Geometry: final body of the model. Coordinates: model frame, mm. Face numbers are marked on the shaded views. Coordinates: 2 decimals unless noted, no trailing zeros. Write each loop counter-clockwise with the first axis right and the second up, starting at its lowest first coordinate (ties: lowest second). Pieces come first, ordered by that corner, then holes. Notation, with made-up numbers: (89.5, 45) -> (148.5, 45) arc R25 cw to (148.5, 81) -> close; hole circle Ø9 at (-23, 47.25). An arc over 180 degrees is marked (long way). Answer as a JSON object with one key per item and string values. Group by question number.
```python
from build123d import *

# Parameters (mm, degrees)
F0_R     = 5
F1_DEPTH = 1
F3_DEPTH = 5
F4_W     = 11.32601
F4_H     = 3.74272
F5_DEPTH = 5
F6_R     = 2.25
F7_DEPTH = 3
F8_R     = 1
F9_DEPTH = 25


with BuildPart() as f1:
    # F0 (on Front) → F1 (new body)
    with BuildSketch(Plane.XZ):
        Circle(F0_R)
    extrude(amount=F1_DEPTH)

    # F2 (on face) → F3 (join)
    with BuildSketch(Plane.XZ.offset(1)):
        with BuildLine():
            ThreePointArc((0, -6), (4.242641, -4.242641), (6, 0))
            ThreePointArc((6, 0), (4.242641, 4.242641), (0, 6))
            ThreePointArc((0, 6), (-3.774917, 4.66369), (-5.868347, 1.25))
            Line((-5.868347, 1.25), (4, 1.25))
            Line((4, 1.25), (4, -1.25))
            Line((4, -1.25), (-5.868347, -1.25))
            ThreePointArc((-5.868347, -1.25), (-3.774917, -4.66369), (0, -6))
        make_face()
        with BuildLine():
            ThreePointArc((-5.868347, 1.25), (-3.774917, 4.66369), (0, 6))
            ThreePointArc((0, 6), (-8.408096, 4.999638), (-16, 1.25))
            Line((-16, 1.25), (-5.868347, 1.25))
        make_face()
        with BuildLine():
            ThreePointArc((-16, -1.25), (-8.408096, -4.999638), (0, -6))
            ThreePointArc((0, -6), (-3.774917, -4.66369), (-5.868347, -1.25))
            Line((-5.868347, -1.25), (-16, -1.25))
        make_face()
        with BuildLine():
            ThreePointArc((-6, 0), (-5.966996, 0.628457), (-5.868347, 1.25))
            Line((-5.868347, 1.25), (-16, 1.25))
            Line((-16, 1.25), (-16, 0))
            Line((-16, 0), (-6, 0))
        make_face()
        with BuildLine():
            Line((-16, -1.25), (-5.868347, -1.25))
            ThreePointArc((-5.868347, -1.25), (-5.966996, -0.628457), (-6, 0))
            Line((-6, 0), (-16, 0))
            Line((-16, 0), (-16, -1.25))
        make_face()
    extrude(amount=F3_DEPTH)

    # F4 (on face) → F5 (join)
    with BuildSketch(Plane.XZ.offset(6)):
        with Locations((-1.024707, -0.007552)):
            Rectangle(F4_W, F4_H)
    extrude(amount=-F5_DEPTH)

    # F6 (on face) → F7 (cut)
    with BuildSketch(Plane(origin=(0, 0, 0), x_dir=(-1, 0, 0), z_dir=(0, 1, 0))):
        Circle(F6_R)
    extrude(amount=-F7_DEPTH, mode=Mode.SUBTRACT)

    # F8 (on face) → F9 (cut)
    with BuildSketch(Plane.XZ.offset(6)):
        Circle(F8_R)
    extrude(amount=-F9_DEPTH, mode=Mode.SUBTRACT)


solid = f1.part
```
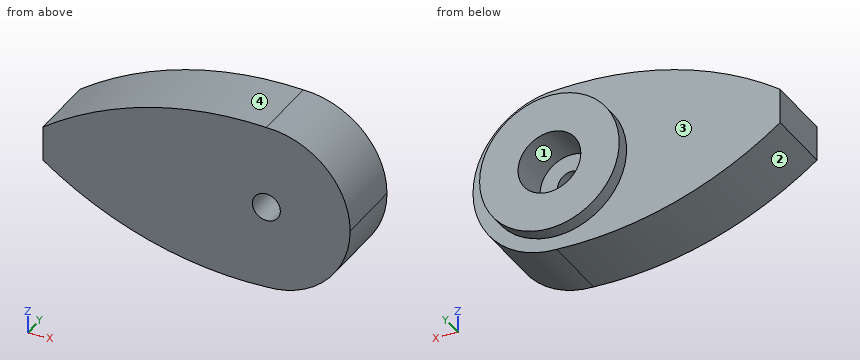
Item 1: Ray query, L1, parallel to Y at x = -10.5, z = -1.5; L2, parallel to X at y = -4.2, z = 0.5; L3, parallel to Y at x = 1.25, z = -1.75. Return the intervals inside material, ascending. Write a range as [from, to].
Item 2: Mould query, pull axis Z, two halves, no side actions, for the marked faces 1, 2, 3 and 4. Classes: +Z half, -Z half, draft (parallel to the pull), parting line (faces both ways), or undercut.
Item 3: Section D-D on x = 1.25. Output: boundary loops of the cut face in (y, z), then the cut area to 3 significant figures.
Item 4: Contact query for flat-ended pins moving along their axis: pin 1 (6 mm diameter, centred on x = -12.5, z = 0, fed in from +Y); pin 2 (4 mm diameter, centred on x = 2.5, z = 3, fed in from +Y); pin 3 (2 mm diameter, centred on y = -2.5, z = -2.5, fed in from -X); pin 4 (2 mm diameter, centred on y = -4.5, z = -4, fed in from +X). Output: stop coordinate, or through.
Item 5: Section A-A on y = -4.5. Output: boundary loops of the cut face in (x, z).
Item 6: Section C-C on y = -1.75. Output: boundary loops of the cut face in (x, z), then the cut area to 3 significant figures.
Item 7: Section B-B on x = -1.75. Output: boundary loops of the cut face in (y, z).
Answer sheet:
{
 "1": {"L1": "y = [-6, -1]", "L2": "x = [-16, -0.87], [0.87, 5.98]", "L3": "y = [-6, -3]"},
 "2": {"face 1": "undercut", "face 2": "-Z half", "face 3": "draft", "face 4": "+Z half"},
 "3": {"outline": "(-6, -5.87) -> (-1, -5.87) -> (-1, -4.84) -> (0, -4.84) -> (0, -1.87) -> (-3, -1.87) -> (-3, 1.87) -> (0, 1.87) -> (0, 4.84) -> (-1, 4.84) -> (-1, 5.87) -> (-6, 5.87) -> close", "area": "57.1 mm^2"},
 "4": {"pin 1": "stops at y = -1", "pin 2": "stops at y = 0", "pin 3": "stops at x = -15.65", "pin 4": "stops at x = 5.2"},
 "5": {"outline": "(-16, -1.25) arc R25 ccw to (0, -6) arc R6 ccw to (6, 0) arc R6 ccw to (0, 6) arc R25 ccw to (-16, 1.25) -> close; hole circle Ø2 at (0, 0)"},
 "6": {"outline": "(-16, -1.25) arc R25 ccw to (0, -6) arc R6 ccw to (6, 0) arc R6 ccw to (0, 6) arc R25 ccw to (-16, 1.25) -> close; hole circle Ø4.5 at (0, 0)", "area": "189 mm^2"},
 "7": {"outline": "(-6, -6.03) -> (-1, -6.03) -> (-1, -4.68) -> (0, -4.68) -> (0, -1.41) -> (-3, -1.41) -> (-3, 1.41) -> (0, 1.41) -> (0, 4.68) -> (-1, 4.68) -> (-1, 6.03) -> (-6, 6.03) -> close"}
}
